Read the model definition and answer for the solid it produces. Units are mm, in the model's axes. A direction names the side the tool comes from. Give positions to 0.01 mm unless a question says otherwise; leave off trailing zeros. Order: outer loops, then holes, each group sorted by start corner. A loop starts at its lowest first (then second) coordinate and runs counter-clockwise, first axis right, second up. Notation, with made-up numbers: (68.5, 11) - (76.5, 11) arc R32 cw to (76.5, 50) - close; hole circle Ø7 at (78.25, -10.75). An arc over 180 degrees is marked (long way). Use a Markdown table: item, result. Add a question column.
1. A cutting plane is placed at B-B on y = 23.5. Determine the outline of the cut face in (x, z), and give its area (3 significant figures).
2. Consider L1, parallel to X at y = 6.1, z = 8; L2, parallel to X at y = 22, z = 5; L3, parallel to X at y = 33, z = 7.5. Determine where each line is inside the solid, lowest interval first.
3. A cutting plane is placed at C-C on z = 4.5. Determine the outline of the cut face in (x, y), and give its area (3 significant figures).
4. Which of the six approach directions +Z, -Z, +X, -X, +Y, -Y give full straight-line access (tool end or side, diameter ignored) to faces 1 (the flat face through (-4.272, 30, 6)), 2 (the flat face through (5.728, 21, 8)), 3 (the flat face through (-17, 7.955, 6))?
5. For a pull along X with two mould halves and no side action, classify faces 4 (the cylindrical face through (15.167, 4.997, 6.731)), 5 (the flat face through (-4, 11, 16)), 6 (the flat face through (17.728, 4, 8)) as released by +X, released by -X, zero draft, split by the parting line, or undercut.
6. Flat-ended cylindrical pins translate along their axes: P1, Ø4, axis at y = 30.29, z = 8, coming from the +X side; P2, Ø4.5, axis at y = 31, z = 9.5, coming from the -X side; P3, Ø4.5, axis at x = -19.27, z = 8, coming from the -Y side; P4, Ø8, axis at y = 16.5, z = 10, coming from the +X side. Find the tip coordinate at first contact, or state that the pin passes through.
7. A cutting plane is placed at D-D on y = 31. Determine the outline of the cut face in (x, z).
8. A cutting plane is placed at A-A on x = -1. Determine the outline of the cut face in (y, z).
Autodesk Inventor part; units mm, degrees
ref_plane "YZ Plane" through (0, 0, 0) normal (1, 0, 0) x (0, 1, 0)
ref_plane "XZ Plane" through (0, 0, 0) normal (0, 1, 0) x (-1, 0, 0)
ref_plane "XY Plane" through (0, 0, 0) normal (0, 0, 1) x (1, 0, 0)
sketch "Esboço1" plane through (0, 0, 0) normal (0, 0, 1) x (1, 0, 0)
  line L0 (17.7277, 1.9549) -> (-24.2723, 1.9549)
  line L1 (-24.2723, 1.9549) -> (-24.2723, 7.9549)
  line L2 (17.7277, 7.9549) -> (17.7277, 1.9549)
  line L3 (5.7277, 34.7549) -> (5.7277, 7.9549)
  line L4 (-12.2723, 7.9549) -> (-12.2723, 34.7549)
  arc A0 (-4.2723, 25.8279) -> (-2.2723, 25.8279) centre (-3.2723, 21.9549) ccw
  line L5 (-24.2723, 7.9549) -> (-12.2723, 7.9549)
  line L6 (5.7277, 7.9549) -> (17.7277, 7.9549)
  line L7 (-2.2723, 34.7549) -> (-2.2723, 25.8279)
  line L8 (-4.2723, 25.8279) -> (-4.2723, 34.7549)
  line L9 (-12.2723, 34.7549) -> (-4.2723, 34.7549)
  line L10 (-2.2723, 34.7549) -> (5.7277, 34.7549)
  dimension "largura" = 42
  dimension "largura_topo" = 18
  dimension "altura_base" = 6
  dimension "diametro" = 8
  dimension "altura_furo" = 20
  dimension "d6" = 12
  dimension "d7" = 9
  dimension "d8" = 6
  dimension "d10" = 8
  dimension "d11" = 8
  dimension "altura" = 32.8
  dimension "d33" = 32.8
extrude "Extrusão1" add sketch "Esboço1" along normal blind 16
sketch "Esboço2" plane through (5.7277, 7.9549, 0) normal (1, 0, 0) x (0, 0, -1)
  line L0 (0, 17.873) -> (-16, 17.873)
  line L1 (-8, 17.873) -> (-8, 26.8) construction
  circle A0 centre (-8, 22.3365) radius 1.1711 construction
  line L2 (0, 26.8) -> (-16, 26.8)
  point P0 (0, -7.9549)
hole "Furo1" at (5.7277, 30.2914, 8) direction (-1, 0, 0) diameter 3.242 end through all counterbore diameter 6 counterbore depth 4
sketch "Esboço3" plane through (-24.2723, 1.9549, 0) normal (0, -1, 0) x (1, 0, 0)
  line L0 (5, 8) -> (37, 8) construction
  circle A0 centre (5, 8) radius 1 construction
  circle A1 centre (37, 8) radius 1 construction
  line L1 (42, 0) -> (0, 0) construction
  line L2 (21, 0) -> (21, 16) construction
  line L3 (0, 16) -> (42, 16) construction
  point P0 (21, 8)
  dimension "distancia_parafusos" = 32
  dimension "d22" = 2
  dimension "d23" = 2
hole "Furo2" at (-19.2723, 1.9549, 8) at (12.7277, 1.9549, 8) direction (0, 1, 0) diameter 5.5 end through all
fillet "Arredondamento1" radius 1 4 edges at (5.7277, 34.7549, 8) (-12.2723, 34.7549, 8) (-24.2723, 7.9549, 8) (17.7277, 7.9549, 8)
equation "\"d6\" = -0.5 * largura_topo + 0.5 * largura"
equation "\"d7\" = 0.5 * largura_topo"
equation "\"d8\" = altura_base"
equation "\"d11\" = d10"
equation "\"d33\" = altura"
properties part number "Sk8"
Output values:
| question | item | result |
|---|---|---|
| 1 | outline | (-12.27, 0) - (-6.96, 0) - (-6.96, 16) - (-12.27, 16) - close; (0.42, 0) - (5.73, 0) - (5.73, 16) - (0.42, 16) - close |
| 1 | area | 170 mm² |
| 2 | L1 | -24.27 to -22.02, -16.52 to 9.98, 15.48 to 17.73 |
| 2 | L2 | -12.27 to -7.27, 0.73 to 5.73 |
| 2 | L3 | -12.27 to -4.27, -2.27 to 1.73 |
| 3 | outline | (-24.27, 1.95) - (17.73, 1.95) - (17.73, 6.95) arc R1 ccw to (16.73, 7.95) - (5.73, 7.95) - (5.73, 33.75) arc R1 ccw to (4.73, 34.75) - (-2.27, 34.75) - (-2.27, 25.83) arc R4 cw (long way) to (-4.27, 25.83) - (-4.27, 34.75) - (-11.27, 34.75) arc R1 ccw to (-12.27, 33.75) - (-12.27, 7.95) - (-23.27, 7.95) arc R1 ccw to (-24.27, 6.95) - close |
| 3 | area | 666 mm² |
| 4 | face 1 | +Z, -Z, +Y |
| 4 | face 2 | +Z, -Z, +X, +Y |
| 4 | face 3 | +Z, -Z, -X, +Y |
| 5 | face 4 | undercut |
| 5 | face 5 | zero draft |
| 5 | face 6 | released by +X |
| 6 | P1 | x = 1.73 |
| 6 | P2 | x = -12.27 |
| 6 | P3 | through |
| 6 | P4 | x = 5.73 |
| 7 | outline | (-12.27, 0) - (-4.27, 0) - (-4.27, 6.54) - (-12.27, 6.54) - close; (-12.27, 9.46) - (-4.27, 9.46) - (-4.27, 16) - (-12.27, 16) - close; (-2.27, 0) - (5.73, 0) - (5.73, 5.08) - (1.73, 5.08) - (1.73, 6.54) - (-2.27, 6.54) - close; (-2.27, 9.46) - (1.73, 9.46) - (1.73, 10.92) - (5.73, 10.92) - (5.73, 16) - (-2.27, 16) - close |
| 8 | outline | (1.95, 0) - (18.66, 0) - (18.66, 16) - (1.95, 16) - close; (25.25, 0) - (34.75, 0) - (34.75, 16) - (25.25, 16) - close; hole circle Ø3.24 at (30.29, 8) |
